Model file for the job. Use its own axes, mm. A direction names the side the tool comes from. Give positions to 0.01 mm unless a question says otherwise; leave off trailing zeros. Write each loop counter-clockwise with the first axis right and the second up, starting at its lowest first coordinate (ties: lowest second). Pieces come first, ordered by that corner, then holes.
```python
from build123d import *

# Parameters (mm, degrees)
SKETCH1_R                = 27.5
BOSS_EXTRUDE1_DEPTH      = 44
BOSS_EXTRUDE1_DEPTH_BACK = 31
CUT_EXTRUDE1_DEPTH       = 10


with BuildPart() as part:
    # Sketch1 → Boss-Extrude1 (new body, two sides)
    with BuildSketch(Plane.XY) as boss_extrude1_sk:
        with Locations((0, -206.1)):
            Circle(SKETCH1_R)
    extrude(amount=BOSS_EXTRUDE1_DEPTH)
    extrude(boss_extrude1_sk.sketch, amount=-BOSS_EXTRUDE1_DEPTH_BACK)

    # Sketch2 → Cut-Extrude1 (cut)
    with BuildSketch(Plane(origin=(0, 0, -31), x_dir=(-1, 0, 0), z_dir=(0, 0, -1))):
        Polygon((22.5, -206.1), (5.5, -191.1), (5.5, -201.1), (-19.5, -201.1), (-19.5, -211.1), (5.5, -211.1), (5.5, -221.1), align=None)
    extrude(amount=-CUT_EXTRUDE1_DEPTH, mode=Mode.SUBTRACT)


solid = part.part
```
1. Slice it at C-C, the plane z = 17. Write the cut outline in (x, y).
Calculated:
outline: circle Ø55 at (0, -206.1)
2. Slice it at A-A, the plane x = 0. Write the cut outline in (y, z), and give its area (4 significant figures).
Calculated:
outline: (-233.6, -31) - (-211.1, -31) - (-211.1, -21) - (-201.1, -21) - (-201.1, -31) - (-178.6, -31) - (-178.6, 44) - (-233.6, 44) - close
area: 4,025 mm2
3. Slice it at D-D, the plane x = 22. Write the cut outline in (y, z), and give its area (4 significant figures).
Calculated:
outline: (-222.6, -31) - (-189.6, -31) - (-189.6, 44) - (-222.6, 44) - close
area: 2,475 mm2
4. Which spindle directions (+Z, -Z, +X, -X, +Y, -Y) get a long thin tool onto all of the face, cutting with end or side? Do faces 4 (the flat face through (0, -206, 44)), 5 (the flat face through (7, -201.1, -26)). Say none if no direction does.
Calculated:
face 4: +Z, +X, -X, +Y, -Y
face 5: -Z
5. Pin check, flat tips, straight feed: P1, Ø5, axis at x = -3, y = -208, coming from the -Z side; P2, Ø8, axis at y = -188, z = 7, coming from the -X side; P3, Ø4, axis at y = -225, z = 1, coming from the +X side. Stop position of each tip, or through.
Calculated:
P1: stops at z = -21
P2: stops at x = -23.61
P3: stops at x = 21.69
6. Slice it at B-B, the plane y = -195. Write the cut outline in (x, z), and give its area (3 significant figures).
Calculated:
outline: (-25.16, -31) - (-9.92, -31) - (-9.92, -21) - (-5.5, -21) - (-5.5, -31) - (25.16, -31) - (25.16, 44) - (-25.16, 44) - close
area: 3,730 mm2
7. Pull direction Y, two halves, no side cores. Call faces 1 (the flat face through (7, -211.1, -26)), 2 (the cylindrical face through (-5.961, -232.946, 7.025)), 3 (the flat face through (0, -212, -31)): +Y half, -Y half, draft (parallel to the pull), parting line (faces both ways), or undercut.
Calculated:
face 1: undercut
face 2: parting line
face 3: draft
8. Probe probe 1 along Y at (x, z) = (-1, 32); probe 2 along Z at (x, y) = (-18, -207); probe 3 along X at (y, z) = (-219, -21.5). List the from-to ranges inside material, lowest first.
Calculated:
probe 1: y = -233.58 to -178.62
probe 2: z = -21 to 44
probe 3: x = -24.29 to -7.88, -5.5 to 24.29
